Could you check a few things on this model? Use its own coordinates, in mm. A direction names the side the tool comes from. Give positions to 0.01 mm unless a question says otherwise; leave off trailing zeros. Loops run counter-clockwise (first coordinate to the right, second up) from the corner with the lowest first, then second, coordinate; pieces in that order, holes last. Notation, with made-up numbers: M 53,-28.75 L 93,-28.75 A26 cw 93,10.25 Z; hole C 33.25,51 d8. An arc over 180 degrees is marked long. Write each question's results on one line, items separated by ' | '. Start each with the question number.
from build123d import *

# Parameters (mm, degrees)
EXTRUDE_START        = -3.2
EXTRUDE_1_DEPTH      = 3.2
SKETCH_2_3_OUTSIDE_W = 47.018
SKETCH_2_3_OUTSIDE_H = 48.224
SKETCH_2_3_OUTSIDE_R = 3.9
CUT_EXTRUDE_2_DEPTH  = 10
CUT_EXTRUDE_2_DRAFT  = -60
CUT_EXTRUDE_START    = -3.2
SKETCH_2_4_OUTSIDE_W = 53.646
SKETCH_2_4_OUTSIDE_H = 54.852
SKETCH_2_4_OUTSIDE_R = 3.9
CUT_EXTRUDE_3_DEPTH  = 11.91362431
CUT_EXTRUDE_3_DRAFT  = 60
FILLET_1_R           = 0.3
CHAMFER_2_SIZE       = 0.111


with BuildPart() as part:
    # 草图1 → 旋转1 (revolve)
    with BuildSketch(Plane.XY, mode=Mode.PRIVATE) as revolve_1_sk:
        Polygon((3.8, 4.9), (2.5, 4.9), (2.5, 0), (3.9, 0), (3.9, 3.2), (3.8, 3.2), align=None)
    revolve(revolve_1_sk.sketch.rotate(Axis((0, 0, 0), (0, 1, 0)), 90), axis=Axis((0, 0, 0), (0, 1, 0)))

    # 草图2 → 凸台-拉伸1 (add)
    with BuildSketch(Plane.XZ.offset(EXTRUDE_START)):
        with BuildLine():
            Line((1.950000027, 3.377499059), (0, 4.5033321))
            Line((0, 4.5033321), (-1.949999961, 3.377499097))
            ThreePointArc((-1.949999961, 3.377499097), (3.8e-08, 3.9), (1.950000027, 3.377499059))
        make_face()
        with BuildLine():
            ThreePointArc((-3.9, 0), (-3.377499063, 1.95000002), (-1.949999961, 3.377499097))
            Line((-1.949999961, 3.377499097), (-3.9, 2.25166605))
            Line((-3.9, 2.25166605), (-3.9, 0))
        make_face()
        with BuildLine():
            Line((3.9, 2.25166605), (1.950000027, 3.377499059))
            ThreePointArc((1.950000027, 3.377499059), (3.377499083, 1.949999986), (3.9, 0))
            Line((3.9, 0), (3.9, 2.25166605))
        make_face()
        with BuildLine():
            ThreePointArc((-1.950000108, -3.377499013), (-3.377499106, -1.949999946), (-3.9, 0))
            Line((-3.9, 0), (-3.9, -2.25166605))
            Line((-3.9, -2.25166605), (-1.950000108, -3.377499013))
        make_face()
        with BuildLine():
            Line((3.9, -2.25166605), (3.9, 0))
            ThreePointArc((3.9, 0), (3.377499044, -1.950000054), (1.949999892, -3.377499137))
            Line((1.949999892, -3.377499137), (3.9, -2.25166605))
        make_face()
        with BuildLine():
            ThreePointArc((1.949999892, -3.377499137), (-1.25e-07, -3.9), (-1.950000108, -3.377499013))
            Line((-1.950000108, -3.377499013), (0, -4.5033321))
            Line((0, -4.5033321), (1.949999892, -3.377499137))
        make_face()
    extrude(amount=EXTRUDE_1_DEPTH)


with BuildPart() as cut_extrude_2_tool:
    # 草图2<3> outside → 切除-拉伸2 (with draft: the straight prism first)
    with BuildSketch(Plane.XZ):
        Rectangle(SKETCH_2_3_OUTSIDE_W, SKETCH_2_3_OUTSIDE_H)
        Circle(SKETCH_2_3_OUTSIDE_R, mode=Mode.SUBTRACT)
    extrude(amount=-CUT_EXTRUDE_2_DEPTH)
    # 切除-拉伸2: the draft: its side faces are tilted about the plane it starts from
    cut_extrude_2_sides = [cut_extrude_2_tool.faces().sort_by_distance(p)[0] for p in [
        (0, 5, -24.112),
        (23.509, 5, 0),
        (0, 5, 24.112),
        (-23.509, 5, 0),
        (-3.9, 5, 0),
    ]]
    draft(cut_extrude_2_sides, Plane.XZ, CUT_EXTRUDE_2_DRAFT)


with BuildPart() as part_1:
    add(part.part)

    # 切除-拉伸2: cut by cut_extrude_2_tool
    add(cut_extrude_2_tool.part, mode=Mode.SUBTRACT)


with BuildPart() as cut_extrude_3_tool:
    # 草图2<4> outside → 切除-拉伸3 (with draft: the straight prism first)
    with BuildSketch(Plane.XZ.offset(CUT_EXTRUDE_START)):
        Rectangle(SKETCH_2_4_OUTSIDE_W, SKETCH_2_4_OUTSIDE_H)
        Circle(SKETCH_2_4_OUTSIDE_R, mode=Mode.SUBTRACT)
    extrude(amount=CUT_EXTRUDE_3_DEPTH)
    # 切除-拉伸3: the draft: its side faces are tilted about the plane it starts from
    cut_extrude_3_sides = [cut_extrude_3_tool.faces().sort_by_distance(p)[0] for p in [
        (0, -2.756812155, -27.426),
        (26.823, -2.756812155, 0),
        (0, -2.756812155, 27.426),
        (-26.823, -2.756812155, 0),
        (-3.9, -2.756812155, 0),
    ]]
    draft(cut_extrude_3_sides, Plane.XZ.offset(CUT_EXTRUDE_START), CUT_EXTRUDE_3_DRAFT)


with BuildPart() as part_2:
    add(part_1.part)

    # 切除-拉伸3: cut by cut_extrude_3_tool
    add(cut_extrude_3_tool.part, mode=Mode.SUBTRACT)

    # 圆角1
    fillet_1_edges = [part_2.edges().sort_by_distance(p)[0] for p in [
        (0, 4.9, 3.8),
    ]]
    fillet(fillet_1_edges, radius=FILLET_1_R)

    # 倒角2
    chamfer_2_edges = [part_2.edges().sort_by_distance(p)[0] for p in [
        (0, 0, 2.5),
        (0, 4.9, 2.5),
    ]]
    chamfer(chamfer_2_edges, length=CHAMFER_2_SIZE)


solid = part_2.part
1) Please list where these lines run through material, in increasing order: line 1 (X direction, y = 3.75, z = 0); line 2 (X direction, y = 2.55, z = 0); line 3 (Y direction, x = -2.5, z = 3). Write a range as from..to.
2) Thinking about a two-plate mould opening in X: for faces 3 (the face through (3.507, 0.083, 2.013)), 4 (the face through (-3.507, 3.117, -2.013)), 5 (the face through (-0.1, 2.4, 2.5)), 6 (the face through (0, 4.9, 3)), which applies, pulls with the +X half, pulls with the -X half, needs draft (parallel to the pull), parting line crosses it, or undercut?
3) Which directions (+Z, -Z, +X, -X, +Y, -Y) give clear straight access to the entire face, cutting with the end or side of a thin tool? Please do faces 1 (the face through (-1.141, 3.91, -3.625)), 2 (the face through (3.497, 3.117, -2.03)).
4) If we section it at B-B on y = 2.45: Write out the boundary of the cut face in (x, z).
5) I'm going to push flat-ended pins straight in: P1, Ø2, axis at y = 4, z = -3, coming from the -X side; P2, Ø1.5, axis at x = 2, y = 0.5, coming from the +Z side. Where does each tip first touch, or does it pass through?
6) If we section it at A-A on y = 3.9: Write out the boundary of the cut face in (x, z).
Calculated:
1) line 1: x = -3.8..-2.5, 2.5..3.8 | line 2: x = -3.9..-2.5, 2.5..3.9 | line 3: y = 0..3.2
2) face 3: pulls with the +X half | face 4: pulls with the -X half | face 5: undercut | face 6: needs draft
3) face 1: +Y | face 2: -Z, +X, +Y
4) outline: M -3.9,-2.25 L 0,-4.5 L 3.9,-2.25 L 3.9,2.25 L 0,4.5 L -3.9,2.25 Z; hole C 0,0 d5
5) P1: stops at x = -3.23 | P2: stops at z = 3.78
6) outline: C 0,0 d7.6; hole C 0,0 d5
